Source: CAD feature listing. Evaluate the final solid. Frame: model axes, mm. Round coordinates to 2 decimals unless told otherwise and drop trailing zeros. Order: outer loops, then holes, each group sorted by start corner. A loop starts at its lowest first (then second) coordinate and runs counter-clockwise, first axis right, second up. Notation, with made-up numbers: (-33.75, -15) - (-9.75, -15) arc R24 ccw to (-9.75, 9) - close; hole circle Ø7 at (70, 3.25). An arc over 180 degrees is marked (long way). Put each result on its own line as item: value. Start each with the question number.
1) Section A-A on y = 0. Output: boundary loops of the cut face in (x, z), then the cut area to 3 significant figures.
2) Contact query for flat-ended pins moving along their axis: P1, Ø2, axis at x = -20.5, z = 1, coming from the +Y side; P2, Ø2, axis at x = -9.5, z = 3, coming from the -Y side; P3, Ø1, axis at y = 24, z = 2.5, coming from the -X side. Output: stop coordinate, or through.
3) Section D-D on x = 17. Output: boundary loops of the cut face in (y, z).
4) Section B-B on x = 0. Output: boundary loops of the cut face in (y, z), then the cut area to 4 significant figures.
5) Line query: probe 1 along Y at (x, z) = (0, 2.8); probe 2 along X at (y, z) = (-0.5, 1.6); probe 3 along X at (y, z) = (9, 0.5). Output: solid intervals per line, ascending. Write a range as [from, to].
6) Section C-C on z = 3.5. Output: boundary loops of the cut face in (x, y), then the cut area to 3 significant figures.
7) Mould query, pull axis Y, two halves, no side actions, for faces 1 (the face through (-21.65, -23.97, 2.54)), 2 (the face through (16, 18, 5)), 3 (the face through (22.37, -7.04, 2.46)). Classes: +Y half, -Y half, draft (parallel to the pull), parting line (faces both ways), or undercut.
Autodesk Inventor part; units mm, degrees
ref_plane "YZ Plane" through (0, 0, 0) normal (1, 0, 0) x (0, 1, 0)
ref_plane "XZ Plane" through (0, 0, 0) normal (0, 1, 0) x (-1, 0, 0)
ref_plane "XY Plane" through (0, 0, 0) normal (0, 0, 1) x (1, 0, 0)
sketch "スケッチ1" plane through (0, 0, 0) normal (0, 0, 1) x (1, 0, 0)
  circle A0 centre (0, 0) radius 23.45
  circle A1 centre (0, 0) radius 36.55
  line L0 (0, 0) -> (-28.1908, 10.2606) construction
  line L1 (0, 0) -> (28.1908, 10.2606) construction
  line L2 (-39.5959, 0) -> (43.1917, 0) construction
  line L3 (0, 0) -> (0, 30) construction
  circle A2 centre (-28.1908, 10.2606) radius 2.55
  circle A3 centre (0, 30) radius 2.55
  circle A4 centre (28.1908, 10.2606) radius 2.55
  dimension "d0" = 73.1
  dimension "d1" = 46.9
  dimension "d2" = 30
  dimension "d3" = 30
  dimension "d6" = 20
  dimension "d7" = 20
  dimension "d8" = 30
  dimension "d9" = 5.1
  dimension "d10" = 5.1
  dimension "d11" = 5.1
extrude "押し出し1" add sketch "スケッチ1" along normal blind 5
sketch "スケッチ2" plane through (0, 0, 5) normal (0, 0, 1) x (1, 0, 0)
  line L0 (0, 0) -> (0, -80) construction
  circle A0 centre (0, -80) radius 52.5
  dimension "d14" = 80
  dimension "d18" = 105
extrude "押し出し2" cut sketch "スケッチ2" against normal blind 10
sketch "スケッチ3" plane through (0, 0, 5) normal (0, 0, 1) x (1, 0, 0)
  circle A0 centre (28.1908, 10.2606) radius 2.55
  line L0 (0, 0) -> (28.1908, 10.2606)
  circle A1 centre (-28.1908, 10.2606) radius 2.55
  line L1 (-28.1908, 10.2606) -> (0, 0)
  circle A2 centre (0, 30) radius 2.55
  line L2 (0, 0) -> (0, 30)
sketch "スケッチ4" plane through (0, 0, 5) normal (0, 0, 1) x (1, 0, 0)
  arc A0 (19.1643, -31.1228) -> (-19.1643, -31.1228) centre (0, 0) ccw
  line L0 (-31.0967, -19.2067) -> (-11.9326, -28.874)
  arc A1 (19.1643, -31.1228) -> (-19.1643, -31.1228) centre (0, -80) ccw
  line L1 (-31.0967, -19.2067) -> (-38.9528, -25.1507)
  line L2 (-38.9528, -25.1507) -> (-33.0141, -34.3769)
  line L3 (-33.0141, -34.3769) -> (-12.5468, -31.9378)
  line L4 (-12.5468, -31.9378) -> (-11.9326, -28.874)
  line L5 (-31.0967, -19.2067) -> (-11.9326, -28.874)
  line L6 (-29.2537, -31.1228) -> (-31.0967, -19.2067)
extrude "押し出し3" cut sketch "スケッチ4" against normal blind 10 contours L0 A1 A0 picked at (-23.5945, -23.9544)
properties part number "円 46.9mm" material "アルミニウム 6061"
Answer sheet:
1. outline: (-36.55, 0) - (-23.45, 0) - (-23.45, 5) - (-36.55, 5) - close; (23.45, 0) - (36.55, 0) - (36.55, 5) - (23.45, 5) - close
1. area: 131 mm^2
2. P1: y = 30.91
2. P2: y = -28.56
2. P3: x = -27.99
3. outline: (-30.33, 0) - (-16.15, 0) - (-16.15, 5) - (-30.33, 5) - close; (16.15, 0) - (32.36, 0) - (32.36, 5) - (16.15, 5) - close
4. outline: (-27.5, 0) - (-23.45, 0) - (-23.45, 5) - (-27.5, 5) - close; (23.45, 0) - (27.45, 0) - (27.45, 5) - (23.45, 5) - close; (32.55, 0) - (36.55, 0) - (36.55, 5) - (32.55, 5) - close
4. area: 60.25 mm^2
5. probe 1: [-27.5, -23.45], [23.45, 27.45], [32.55, 36.55]
5. probe 2: [-36.55, -23.44], [23.44, 36.55]
5. probe 3: [-35.42, -30.41], [-25.97, -21.65], [21.65, 25.97], [30.41, 35.42]
6. outline: (-31.1, -19.21) - (-11.93, -28.87) arc R52.5 cw to (19.16, -31.12) arc R36.55 ccw (long way) to start; hole circle Ø5.1 at (-28.19, 10.26); hole circle Ø46.9 at (0, 0); hole circle Ø5.1 at (0, 30); hole circle Ø5.1 at (28.19, 10.26)
6. area: 2,110 mm^2
7. face 1: -Y half
7. face 2: draft
7. face 3: undercut
